Autodesk Inventor part; units mm, degrees
ref_plane "YZ Plane" through (0, 0, 0) normal (1, 0, 0) x (0, 1, 0)
ref_plane "XZ Plane" through (0, 0, 0) normal (0, 1, 0) x (-1, 0, 0)
ref_plane "XY Plane" through (0, 0, 0) normal (0, 0, 1) x (1, 0, 0)
sketch "Sketch3" plane through (0, 0, 0) normal (0, 0, 1) x (1, 0, 0)
  circle A0 centre (0, 0) radius 2
  line L0 (0, 0) -> (12.75, 0)
  line L1 (12.75, 0) -> (12.75, -26)
  line L2 (12.75, -26) -> (4.75, -26)
  line L3 (4.75, -26) -> (4.75, -16)
  circle A1 centre (0, 0) radius 12.75
  line L4 (4.75, -16) -> (4.75, 8)
  line L5 (4.75, 8) -> (12.75, 8)
  line L6 (12.75, 8) -> (12.75, 0)
  circle A2 centre (0, 0) radius 8
  line L7 (0, -8) -> (4.75, -8)
  line L8 (0, 8) -> (4.75, 8)
  dimension "d29" = 4
  dimension "d30" = 12.75
  dimension "d31" = 26
  dimension "d32" = 8
  dimension "d33" = 10
  dimension "d34" = 8
extrude "Extrusion2" add sketch "Sketch3" along normal mid plane 10 contours A2 L4 L5 A1 L0 | A2 L4 L0 | L0 L4 A2 | L0 A1 L4 A2 | L1 L2 L3 L4 A1 | A1 L5 L6 | L4 A2 | A2 L8 L4 | L4 L7 A2
sketch "Sketch4" plane through (12.75, -26, 5) normal (1, 0, 0) x (0, 0, -1)
  line L0 (10, 0) -> (0, 0)
  point P0 (5, 26)
  point P1 (5, 4)
  point P2 (5, 11)
  dimension "d37" = 7
  dimension "d38" = 4
hole "Hole2" at (12.75, -22, 0) at (12.75, -15, 0) direction (-1, 0, 0) diameter 2.459 end through all
properties part number "CHUCKLENGAN"
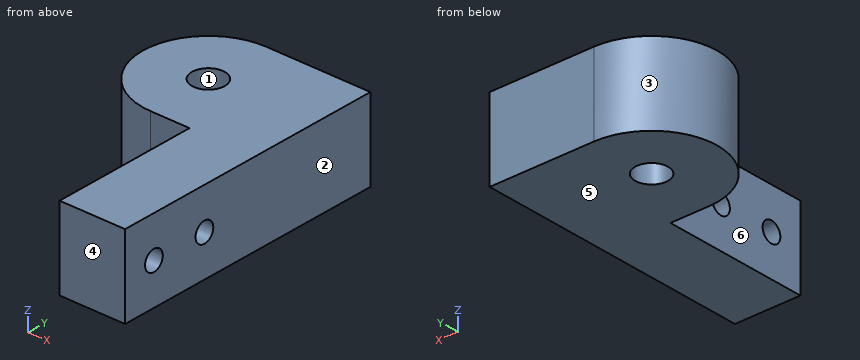
The model under review builds one solid part; all positions refer to its coordinate system, in mm. Face numbers are marked on the shaded views. A direction names the side the tool comes from. Coordinates: 2 decimals unless noted, no trailing zeros. Order: outer loops, then holes, each group sorted by start corner. A loop starts at its lowest first (then second) coordinate and runs counter-clockwise, first axis right, second up. Notation, with made-up numbers: (36, 35.5) -> (90, 35.5) arc R23 ccw to (90, 44.5) -> close; hole circle Ø8 at (-11.5, -26.5). An arc over 180 degrees is marked (long way). Answer in a Markdown table with one row per item.
(1) Consider section C-C (x = 9). Write out the cut boundary in (y, z).
Answers:
| item | result |
|---|---|
| outline | (-26, -5) -> (8, -5) -> (8, 5) -> (-26, 5) -> close; hole circle Ø2.46 at (-22, 0); hole circle Ø2.46 at (-15, 0) |
(2) The part is to be moulded in two halves that separate along X. For the marked faces 1, 2, 3 and 4, say which applies: +X half, -X half, draft (parallel to the pull), parting line (faces both ways), or undercut.
Answers:
| item | result |
|---|---|
| face 1 | undercut |
| face 2 | +X half |
| face 3 | -X half |
| face 4 | draft |
(3) Wall thickness on line 1 along Y through (x, z) = (8.5, 0); line 2 along Z through (x, y) = (7.25, -22); line 3 along Y through (x, z) = (0, -3): over which ranges is each line inside the solid? List them lowest first.
Answers:
| item | result |
|---|---|
| line 1 | -26 to -23.23, -20.77 to -16.23, -13.77 to 8 |
| line 2 | -5 to -1.23, 1.23 to 5 |
| line 3 | -8 to -2, 2 to 8 |
(4) Machinability: for the marked faces 5 and 6, which of the approach directions +Z, -Z, +X, -X, +Y, -Y give a long, thin tool a straight path to every point of the face, cutting with its end or side? Answer none if there is none.
Answers:
| item | result |
|---|---|
| face 5 | -Z, +X, -X, +Y, -Y |
| face 6 | +Z, -Z, -X, -Y |
(5) Consider section D-D (z = 2.5). Write out the cut boundary in (x, y).
Answers:
| item | result |
|---|---|
| outline | (0, -8) -> (4.75, -8) -> (4.75, -26) -> (12.75, -26) -> (12.75, 8) -> (0, 8) arc R8 ccw to start; hole circle Ø4 at (0, 0) |
(6) Consider section A-A (z = 0). Write out the cut boundary in (x, y).
Answers:
| item | result |
|---|---|
| outline | (0, -8) -> (4.75, -8) -> (4.75, -13.77) -> (12.75, -13.77) -> (12.75, 8) -> (0, 8) arc R8 ccw to start; (4.75, -26) -> (12.75, -26) -> (12.75, -23.23) -> (4.75, -23.23) -> close; (4.75, -20.77) -> (12.75, -20.77) -> (12.75, -16.23) -> (4.75, -16.23) -> close; hole circle Ø4 at (0, 0) |
(7) Consider section B-B (y = -22). Write out the cut boundary in (x, z), plus the area to 3 significant figures.
Answers:
| item | result |
|---|---|
| outline | (4.75, -5) -> (12.75, -5) -> (12.75, -1.23) -> (4.75, -1.23) -> close; (4.75, 1.23) -> (12.75, 1.23) -> (12.75, 5) -> (4.75, 5) -> close |
| area | 60.3 mm² |
(8) Insertion check: pin 1 (5 mm diameter, centred on y = -19, z = 3.5, fed in from -X); pin 2 (1 mm diameter, centred on x = 2.5, z = 1, fed in from -Y); pin 3 (5 mm diameter, centred on x = 2, y = -19, fed in from +Z). Each pin has a flat end and moves straight along its axis. Give the tip position at first contact, or say it passes through.
Answers:
| item | result |
|---|---|
| pin 1 | x = 4.75 |
| pin 2 | y = -8 |
| pin 3 | through |
